from build123d import *

# Parameters (mm, degrees)
F0_R      = 254
F1_DEPTH  = 76.2
F2_R      = 88.9
F3_DEPTH  = 152.4
F4_R      = 63.5
F5_DEPTH  = 152.4
F7_R      = 102.731788
F8_DEPTH  = 25.4
F9_R      = 220.675827
F10_DEPTH = 12.7
F6_R      = 15.24
F11_DEPTH = 152.4


with BuildPart() as f1:
    # F0 (on Top) → F1 (new body)
    with BuildSketch(Plane.XY):
        Circle(F0_R)
    extrude(amount=F1_DEPTH)

    # F2 (on face) → F3 (cut)
    with BuildSketch(Plane.XY.offset(76.2)):
        Circle(F2_R)
    extrude(amount=-F3_DEPTH, mode=Mode.SUBTRACT)

    # F4 (on face) → F5 (cut)
    with BuildSketch(Plane.XY.offset(76.2)):
        with Locations((0, 172.72)):
            Circle(F4_R)
        with Locations((136.619191, 105.675896)):
            Circle(F4_R)
        with Locations((167.255145, -43.103538)):
            Circle(F4_R)
        with Locations((-82.586414, -151.69602)):
            Circle(F4_R)
        with Locations((-169.291327, -34.243903)):
            Circle(F4_R)
        with Locations((-139.175909, 102.285213)):
            Circle(F4_R)
        with Locations((65.877814, -159.66312)):
            Circle(F4_R)
    extrude(amount=-F5_DEPTH, mode=Mode.SUBTRACT)

    # F7 (on face) → F8 (cut)
    with BuildSketch(Plane.XY.offset(76.2)):
        Circle(F7_R)
    extrude(amount=-F8_DEPTH, mode=Mode.SUBTRACT)

    # F9 (on face) → F10 (cut)
    with BuildSketch(Plane.XY.offset(76.2)):
        Circle(F9_R)
    extrude(amount=-F10_DEPTH, mode=Mode.SUBTRACT)

    # F6 (on face) → F11 (cut)
    with BuildSketch(Plane.XY.offset(76.2)):
        with Locations((-101.82795, 196.120445)):
            Circle(F6_R)
        with Locations((99.8231, 197.148444)):
            Circle(F6_R)
        with Locations((217.796701, 37.373219)):
            Circle(F6_R)
        with Locations((164.933983, -147.067813)):
            Circle(F6_R)
        with Locations((-180.397614, -127.627823)):
            Circle(F6_R)
        with Locations((-216.110642, 46.134055)):
            Circle(F6_R)
        with Locations((-10.606943, -220.725289)):
            Circle(F6_R)
    extrude(amount=-F11_DEPTH, mode=Mode.SUBTRACT)


solid = f1.part
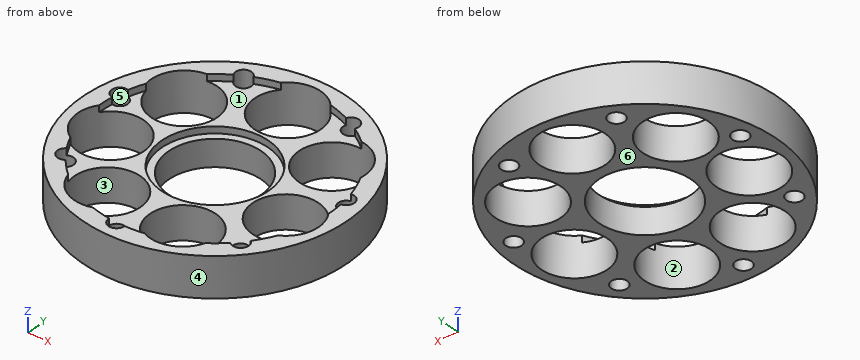
Input: part model. Units: mm. Frame: model coordinates. Face numbers are marked on the shaded views. A direction names the side the tool comes from. Coordinates: 2 decimals unless noted, no trailing zeros. Write each loop counter-clockwise with the first axis right and the second up, starting at its lowest first coordinate (ties: lowest second). Pieces come first, ordered by that corner, then holes. Notation, with made-up numbers: M -37.5,36.5 L 17.5,36.5 A16 ccw 17.5,55.5 Z; hole C 51,73.5 d2. An arc over 180 degrees is marked long. Answer as a JSON object with one key per item and string values. Group by question number.
(1) Contact query for flat-ended pins moving along their axis: P1, Ø8, axis at x = -176.5, z = 44, coming from the -Y side; P2, Ø1.5, axis at x = -49, z = 43, coming from the -Y side; P3, Ø4, axis at x = 21, y = -116, coming from the +Z side. Output: stop coordinate, or through.
(2) Section A-A on x = -156. Output: boundary loops of the cut face in (y, z).
(3) Mould query, pull axis X, two halves, no side actions, for the marked faces 3, 4, 5 and 6. Classes: pulls with the +X half, pulls with the -X half, needs draft (parallel to the pull), parting line crosses it, or undercut.
(4) Section D-D on z = 12.5. Give the number of separate pieces and of enclosed holes in the cut face, plus the area to 3 significant figures.
(5) Set-up query: the marked faces 1 and 2. Return all of +Z, -Z, +X, -X, +Y, -Y with unobstructed straight access to the full face (end or side cutting, diameter ignored); none if empty.
(6) Section B-B on y = -66.5. Output: boundary loops of the cut face in (x, z), plus the area to 3 significant figures.
(7) Ray query, line 1 along Y through (x, z) = (24, 23); line 2 along X through (y, z) = (127, 42); line 3 along Y through (x, z) = (-95, 34). Return the intervals inside material, ascending. Write a range as [from, to].
(8) Section C-C on x = -53.5. Output: boundary loops of the cut face in (y, z), plus the area to 3 significant figures.
Result set:
{
 "1": {"P1": "stops at y = -186.44", "P2": "stops at y = -249.38", "P3": "stops at z = 63.5"},
 "2": {"outline": "M -200.45,0 L -96.34,0 L -96.34,63.5 L -156.08,63.5 L -156.08,76.2 L -200.45,76.2 Z; M 27.85,0 L 41.05,0 L 41.05,63.5 L 27.85,63.5 Z; M 163.52,0 L 200.45,0 L 200.45,76.2 L 163.52,76.2 Z"},
 "3": {"face 3": "undercut", "face 4": "parting line crosses it", "face 5": "undercut", "face 6": "needs draft"},
 "4": {"separate pieces": "1", "enclosed holes": "15", "area": "84,100 mm2"},
 "5": {"face 1": "+Z", "face 2": "+Z, -Z"},
 "6": {"outline": "M -245.14,0 L -223.99,0 L -223.99,76.2 L -245.14,76.2 Z; M -114.59,0 L -59,0 L -59,50.8 L -78.3,50.8 L -78.3,63.5 L -114.59,63.5 Z; M 59,0 L 108.22,0 L 108.22,63.5 L 78.3,63.5 L 78.3,50.8 L 59,50.8 Z; M 226.29,0 L 245.14,0 L 245.14,76.2 L 226.29,76.2 Z", "area": "9,210 mm2"},
 "7": {"line 1": "y = [-252.86, -207.4], [-111.93, -85.6], [85.6, 113.93], [231.51, 252.86]", "line 2": "x = [-219.97, -197.67], [-80.68, -44.07], [44.07, 76.81], [196.43, 219.97]", "line 3": "y = [-235.57, -213.97], [-89.42, 56.67], [147.9, 182.5], [209.75, 235.57]"},
 "8": {"outline": "M -248.3,0 L -208.14,0 L -208.14,63.5 L -214.09,63.5 L -214.09,76.2 L -248.3,76.2 Z; M -95.25,0 L -71,0 L -71,50.8 L -87.7,50.8 L -87.7,63.5 L -95.25,63.5 Z; M 71,0 L 138.51,0 L 138.51,63.5 L 87.7,63.5 L 87.7,50.8 L 71,50.8 Z; M 206.93,0 L 248.3,0 L 248.3,76.2 L 214.09,76.2 L 214.09,63.5 L 206.93,63.5 Z", "area": "11,400 mm2"}
}
